Answer from the drawing. Dimensions are ordinates in mm from the lowest x, y and z of the part. A direction names the side the tool comes from. Round coordinates to 2 decimals unless told otherwise and drop trailing zeros. Write each loop counter-clockwise with the first axis right and the second up, starting at its lowest first coordinate (ties: lowest second). Pieces come first, ordered by that corner, then holes. Notation, with made-up numbers: M 27.5,53.5 L 58.5,53.5 A23 ccw 58.5,67.5 Z; hole C 58,22.25 d3. An arc over 180 degrees is marked long. One line per item, written item: value. Start each with the question number.
(1) Section A-A (x = 7.5) is taken. Determine the outline of the cut face in (y, z).
(2) Given P1, Ø4.5, axis at x = 4.5, y = 10, coming from the -Z side; P2, Ø5, axis at y = 10.5, z = 1.5, coming from the +X side; P3, Ø8, axis at x = 11.5, z = 8.5, coming from the -Y side; P4, Ø1, axis at x = 4.5, z = 1.5, coming from the +Y side, each flat-ended and moving along its own axis, determine where each tip first touches the part or whether it passes through.
(3) Consider probe 1 along Z at (x, y) = (6, 6.75); probe 2 along Z at (x, y) = (13, 7); probe 3 along X at (y, z) = (5, 10). Determine where each line is inside the solid, lowest interval first.
(4) Section D-D (z = 9.5) is taken. Determine the outline of the cut face in (x, y).
(5) For the marked faces 1 and 2, determine the directions among +Z, -Z, +X, -X, +Y, -Y from which every point of the face is accessible in a straight line to the end or side of a thin tool.
(6) Section C-C (z = 5.75) is taken. Determine the outline of the cut face in (x, y), plus the area to 3 significant figures.
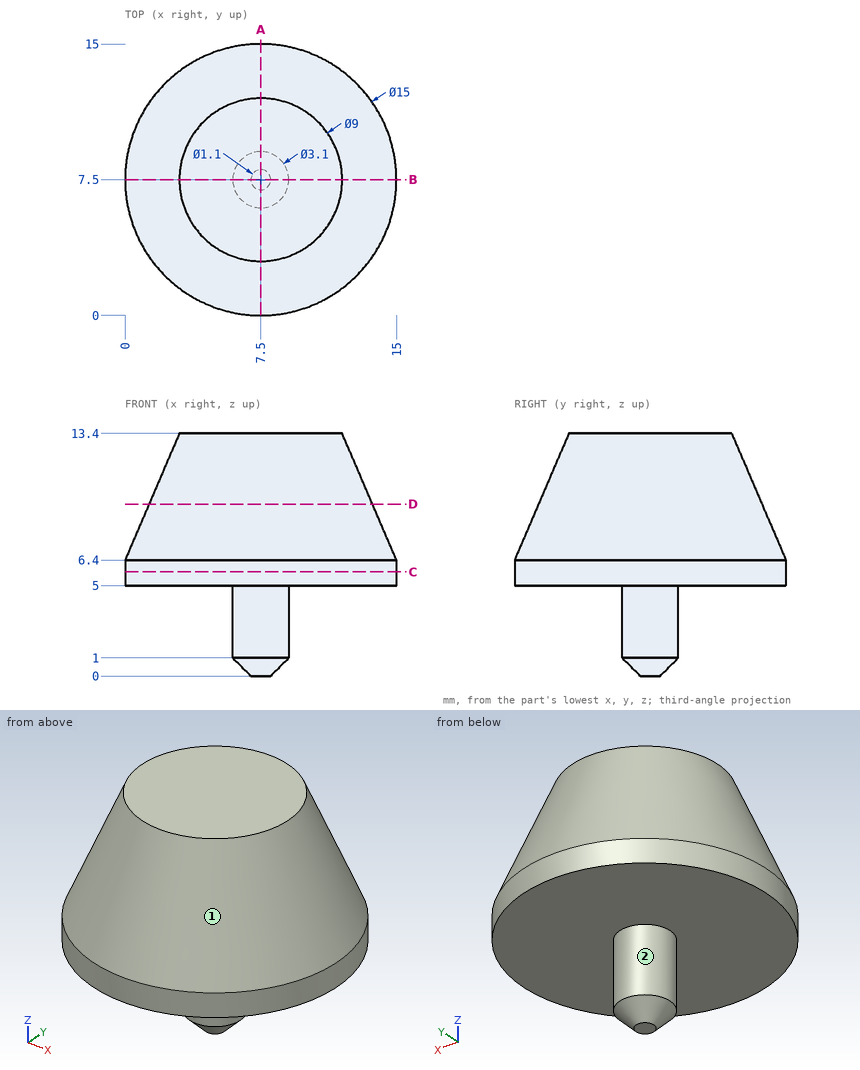
Recorded:
1. outline: M 0,5 L 5.95,5 L 5.95,1 L 6.95,0 L 8.05,0 L 9.05,1 L 9.05,5 L 15,5 L 15,6.4 L 12,13.4 L 3,13.4 L 0,6.4 Z
2. P1: stops at z = 5
2. P2: stops at x = 8.97
2. P3: stops at y = 0.02
2. P4: passes through
3. probe 1: z = 5 to 13.4
3. probe 2: z = 5 to 11.01
3. probe 3: x = 2.09 to 12.91
4. outline: C 7.5,7.5 d12.34
5. face 1: +Z
5. face 2: -Z
6. outline: C 7.5,7.5 d15
6. area: 177 mm2
